from build123d import *

# Parameters (mm, degrees)
SKETCH1_W           = 120
SKETCH1_H           = 76
BOSS_EXTRUDE1_DEPTH = 1.6
SKETCH2_R           = 1.25
CUT_EXTRUDE1_DEPTH  = 72.039144139


with BuildPart() as part:
    # Sketch1 → Boss-Extrude1 (new body)
    with BuildSketch(Plane(origin=(0, 0, 0), x_dir=(1, 0, 0), z_dir=(0, 1, 0))):
        Rectangle(SKETCH1_W, SKETCH1_H)
    extrude(amount=-BOSS_EXTRUDE1_DEPTH)

    # Sketch2 → Cut-Extrude1 (cut, through all)
    with BuildSketch(Plane(origin=(0, 0, 0), x_dir=(1, 0, 0), z_dir=(0, 1, 0))):
        with Locations(Location((-54.5, 32.5, 0), (0, 0, 270))):
            Circle(SKETCH2_R)
        with Locations(Location((-54.5, -32.5, 0), (0, 0, 270))):
            Circle(SKETCH2_R)
        with Locations(Location((33.5, 32.5, 0), (0, 0, 270))):
            Circle(SKETCH2_R)
        with Locations(Location((33.5, -32.5, 0), (0, 0, 270))):
            Circle(SKETCH2_R)
    extrude(amount=-CUT_EXTRUDE1_DEPTH, mode=Mode.SUBTRACT)


solid = part.part
Could you check a few things on this model? Use its own coordinates, in mm. Give positions to 0.01 mm unless a question says otherwise; leave off trailing zeros. Order: outer loops, then holes, each group sorted by start corner. A loop starts at its lowest first (then second) coordinate and runs counter-clockwise, first axis right, second up. Notation, with made-up numbers: (20, 15) - (47, 15) arc R38 ccw to (47, 53) - close; hole circle Ø10 at (38.25, -29). An arc over 180 degrees is marked (long way). One line per question, with ' | ' between items. Start each with the question number.
Item 1: I want a section at B-B on x = 33.5. Write out the boundary of the cut face in (y, z).
Item 2: Thinking about a two-plate mould opening in Z: for faces 1 (the cylindrical face through (32.391, -0.789, -31.923)), 2 (the flat face through (-1, -1.6, -1)), which applies, pulls with the +Z half, pulls with the -Z half, needs draft (parallel to the pull), parting line crosses it, or undercut?
Item 3: I need wall thicknesses on probe 1 along X at (y, z) = (-0.6, -32.5). Which ranges of the line are inside material? Lowest first, please. Write a range as [from, to].
Item 4: I want a section at A-A on z = 32.5. Write out the boundary of the cut face in (x, y).
Verdict:
1) outline: (-1.6, -38) - (0, -38) - (0, -33.75) - (-1.6, -33.75) - close; (-1.6, -31.25) - (0, -31.25) - (0, 31.25) - (-1.6, 31.25) - close; (-1.6, 33.75) - (0, 33.75) - (0, 38) - (-1.6, 38) - close
2) face 1: undercut | face 2: needs draft
3) probe 1: [-60, -55.75], [-53.25, 32.25], [34.75, 60]
4) outline: (-60, -1.6) - (-55.75, -1.6) - (-55.75, 0) - (-60, 0) - close; (-53.25, -1.6) - (32.25, -1.6) - (32.25, 0) - (-53.25, 0) - close; (34.75, -1.6) - (60, -1.6) - (60, 0) - (34.75, 0) - close
